Read the model definition and answer for the solid it produces. Units are mm, in the model's axes. Face numbers are marked on the shaded views. A direction names the side the tool comes from. Give positions to 0.01 mm unless a question says otherwise; leave off trailing zeros. Write each loop counter-clockwise with the first axis right and the second up, starting at its lowest first coordinate (ties: lowest second). Pieces come first, ordered by that corner, then holes.
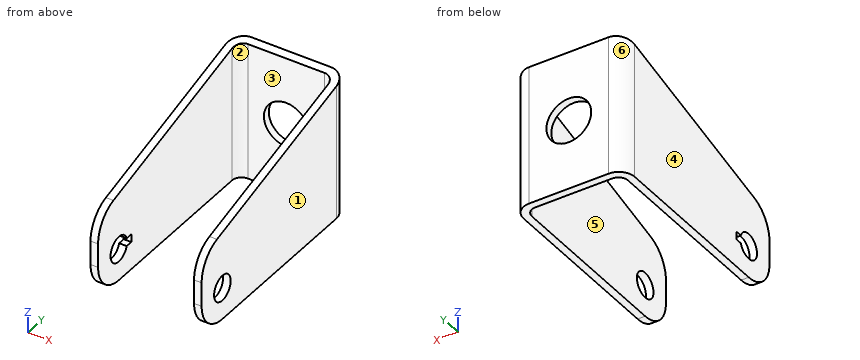
```python
from build123d import *

# Parameters (mm, degrees)
BOSS_EXTRUDE1_DEPTH = 22
CUT_EXTRUDE1_DEPTH  = 18.5
SKETCH4_R           = 4
CUT_EXTRUDE2_DEPTH  = 18.5
FILLET2_R           = 10
FILLET3_R           = 10
SKETCH5_R           = 7.05
CUT_EXTRUDE3_DEPTH  = 71
CUT_EXTRUDE6_REACH  = 37


with BuildPart() as part:
    # Sketch1 → Boss-Extrude1 (new body, symmetric)
    with BuildSketch(Plane.XY):
        with BuildLine():
            Line((0, 0), (12.5, 0))
            ThreePointArc((12.5, 0), (16.035533906, -1.464466094), (17.5, -5))
            Line((17.5, -5), (17.5, -70))
            Line((17.5, -70), (15.12, -70))
            Line((15.12, -70), (15.12, -5.38))
            ThreePointArc((15.12, -5.38), (14.241320344, -3.258679656), (12.12, -2.38))
            Line((12.12, -2.38), (0, -2.38))
            Line((0, -2.38), (0, 0))
        make_face()
    extrude(amount=BOSS_EXTRUDE1_DEPTH, both=True)

    # Sketch3 → Cut-Extrude1 (cut, through all)
    with BuildSketch(Plane(origin=(17.5, 0, 0), x_dir=(0, 0, -1), z_dir=(1, 0, 0))):
        Polygon((-22, 0), (-22, -70), (-3.24355653, -70), align=None)
    extrude(amount=-CUT_EXTRUDE1_DEPTH, mode=Mode.SUBTRACT)

    # Sketch4 → Cut-Extrude2 (cut, through all)
    with BuildSketch(Plane(origin=(17.5, 0, 0), x_dir=(0, 0, -1), z_dir=(1, 0, 0))):
        with Locations((12, -60)):
            Circle(SKETCH4_R)
    extrude(amount=-CUT_EXTRUDE2_DEPTH, mode=Mode.SUBTRACT)

    # Fillet2
    fillet2_edges = [part.edges().sort_by_distance(p)[0] for p in [
        (16.31, -70, -22),
    ]]
    fillet(fillet2_edges, radius=FILLET2_R)

    # Fillet3
    fillet3_edges = [part.edges().sort_by_distance(p)[0] for p in [
        (16.31, -70, 3.24355653),
    ]]
    fillet(fillet3_edges, radius=FILLET3_R)

    # Mirror1: part across plane


with BuildPart() as part_1:
    add(part.part)
    add(part.part.mirror(Plane(origin=(0, 0, 0), x_dir=(0, 0, 1), z_dir=(1, 0, 0))))

    # Sketch5 → Cut-Extrude3 (cut, through all)
    with BuildSketch(Plane(origin=(0, 0, 0), x_dir=(1, 0, 0), z_dir=(0, 1, 0))):
        Circle(SKETCH5_R)
    extrude(amount=-CUT_EXTRUDE3_DEPTH, mode=Mode.SUBTRACT)

    # Sketch7 → Cut-Extrude6 (cut, up to next)
    with BuildSketch(Plane.ZY.offset(17.5), mode=Mode.PRIVATE) as cut_extrude6_sk1:
        Polygon((-13.25, -54), (-10.75, -54), (-10.75, -56.200328962), (-10.75, -56.332123316), (-13.25, -56.332123316), (-13.25, -56.200328962), align=None)
    cut_extrude6_tool1 = extrude(cut_extrude6_sk1.sketch, amount=-CUT_EXTRUDE6_REACH, mode=Mode.PRIVATE) & part_1.part
    add(cut_extrude6_tool1.solids().sort_by_distance((-17.5, -55.166062, -12))[0], mode=Mode.SUBTRACT)


solid = part_1.part
```
Item 1: Find the intervals of material crossed by line 1 along X through (y, z) = (-63.5, -3); line 2 along Y through (x, z) = (9.5, -16); line 3 along X through (y, z) = (-0.9, 0), in increasing order.
Result set:
line 1: x = -17.5 to -15.12, 15.12 to 17.5
line 2: y = -2.38 to 0
line 3: x = -15.36 to -7.05, 7.05 to 15.36
Item 2: Section C-C (z = 0) is taken. Write down the section's boundary in (x, y).
Result set:
outline: (-17.5, -68.97) - (-15.12, -68.97) - (-15.12, -5.38) arc R3 cw to (-12.12, -2.38) - (-7.05, -2.38) - (-7.05, 0) - (-12.5, 0) arc R5 ccw to (-17.5, -5) - close; (7.05, -2.38) - (12.12, -2.38) arc R3 cw to (15.12, -5.38) - (15.12, -68.97) - (17.5, -68.97) - (17.5, -5) arc R5 ccw to (12.5, 0) - (7.05, 0) - close
Item 3: Section A-A (x = 0) is taken. Write down the section's boundary in (y, z), and give its area (3 significant figures).
Result set:
outline: (-2.38, -22) - (0, -22) - (0, -7.05) - (-2.38, -7.05) - close; (-2.38, 7.05) - (0, 7.05) - (0, 22) - (-2.38, 21.36) - close
area: 70.4 mm2
Item 4: Which of the six approach directions +Z, -Z, +X, -X, +Y, -Y give full straight-line access (tool end or side, diameter ignored) to the marked faces 5 and 6?
Result set:
face 5: +Z, -Z, -Y
face 6: +Z, -Z, -X, +Y
Item 5: Section B-B (y = -16) is taken. Write down the section's boundary in (x, z), and give its area (3 significant figures).
Result set:
outline: (-17.5, -22) - (-15.12, -22) - (-15.12, 17.71) - (-17.5, 17.71) - close; (15.12, -22) - (17.5, -22) - (17.5, 17.71) - (15.12, 17.71) - close
area: 189 mm2
Item 6: Section D-D (y = -57) is taken. Write down the section's boundary in (x, z).
Result set:
outline: (-17.5, -22) - (-15.12, -22) - (-15.12, -14.65) - (-17.5, -14.65) - close; (-17.5, -9.35) - (-15.12, -9.35) - (-15.12, 6.73) - (-17.5, 6.73) - close; (15.12, -22) - (17.5, -22) - (17.5, -14.65) - (15.12, -14.65) - close; (15.12, -9.35) - (17.5, -9.35) - (17.5, 6.73) - (15.12, 6.73) - close
Item 7: Each of these flat-tipped pins is pushed along its axis until it touches: pin 1 Ø0.7 at (x, y) = (-17, -55.5) entering from +Z; pin 2 Ø7.5 at (x, z) = (4.5, -4) entering from -Y. Where does it stop, or does it pass through?
Result set:
pin 1: stops at z = 7.22
pin 2: stops at y = -2.38
Item 8: Determine the mould class of the marked faces 1, 2, 3 and 4 for opening direction X: pulls with the +X half, pulls with the -X half, needs draft (parallel to the pull), parting line crosses it, or undercut.
Result set:
face 1: pulls with the +X half
face 2: undercut
face 3: undercut
face 4: pulls with the -X half
